Can you work these out from the model? Positions are in its coordinate system, mm. A direction names the side the tool comes from. Round coordinates to 2 decimals unless told otherwise and drop trailing zeros. Loops run counter-clockwise (first coordinate to the right, second up) from the corner with the lowest first, then second, coordinate; pieces in that order, holes last. Notation, with made-up numbers: M 41.5,-4.5 L 61.5,-4.5 A24 ccw 61.5,16.5 Z; hole C 85.5,-2 d9. An arc over 180 degrees is marked long. Return JSON: item names as keys, results as strings.
Autodesk Inventor part; units mm, degrees
ref_plane "YZ Plane" through (0, 0, 0) normal (1, 0, 0) x (0, 1, 0)
ref_plane "XZ Plane" through (0, 0, 0) normal (0, 1, 0) x (-1, 0, 0)
ref_plane "XY Plane" through (0, 0, 0) normal (0, 0, 1) x (1, 0, 0)
sketch "Esquisse1" plane through (0, 0, 0) normal (0, 0, 1) x (1, 0, 0)
  circle A0 centre (0, 0) radius 3
  dimension "d0" = 6
extrude "Extrusion1" add sketch "Esquisse1" along normal blind 36.5
sketch "Esquisse2" plane through (0, 0, 36.5) normal (0, 0, 1) x (1, 0, 0)
  circle A0 centre (0, 0) radius 2.5
  dimension "d3" = 5
extrude "Extrusion2" add sketch "Esquisse2" along normal blind 3
sketch "Esquisse3" plane through (0, 0, 0) normal (0, 0, -1) x (-1, 0, 0)
  circle A0 centre (0, 0) radius 2.5
  dimension "d6" = 5
extrude "Extrusion3" add sketch "Esquisse3" along normal blind 12
sketch "Esquisse4" plane through (0, 0, -12) normal (0, 0, -1) x (-1, 0, 0)
  circle A0 centre (0, 0) radius 2
  dimension "d9" = 4
extrude "Extrusion4" add sketch "Esquisse4" along normal blind 29
thread "Filetage1"
fillet "Congé1" radius 0.5 1 edges at (2, 0, -41)
properties part number "AxeArriere" material "Acier inoxydable"
Q1. On a 3-axis mill with a long thin cutter (end or side, diameter ignored), from which of +Z, -Z, +X, -X, +Y, -Y can I reach the whole of each face in a straight line? I mean faces 1 (the flat face through (0, 0, -41)), 2 (the cylindrical face through (0.54, 2.44, -5.92)), 3 (the cylindrical face through (-0.54, 2.44, 37.98)). Say none if no direction works.
Results:
{"face 1": "-Z, +X, -X, +Y, -Y", "face 2": "-Z", "face 3": "+Z"}
Q2. Suppose I cut it at C-C, the plane z = -1. Please give me the cut outline in (x, y), plus the area to 3 significant figures.
Results:
{"outline": "C 0,0 d5", "area": "19.6 mm2"}
Q3. Suppose I cut it at D-D, the plane z = -19. Please give me the cut outline in (x, y), plus the area to 3 significant figures.
Results:
{"outline": "C 0,0 d4", "area": "12.6 mm2"}
Q4. If I drill on line 1 along Z through (x, y) = (-0.85, -2.65); line 2 along Z through (x, y) = (1.15, 1.75); line 3 along X through (y, z) = (0.1, 11), over which ranges is the centre line in solid material (lowest first)?
Results:
{"line 1": "z = 0 to 36.5", "line 2": "z = -12 to 39.5", "line 3": "x = -3 to 3"}
Q5. I'm going to push flat-ended pins straight in: pin 1 Ø1.5 at (y, z) = (2, 7.5) entering from +X; pin 2 Ø1 at (x, z) = (0, -22.5) entering from +Y. Where does each tip first touch, or does it pass through?
Results:
{"pin 1": "stops at x = 2.73", "pin 2": "stops at y = 2"}
Q6. Suppose I cut it at A-A, the plane x = 0. Please give me the cut outline in (y, z), plus the area to 3 significant figures.
Results:
{"outline": "M -3,0 L -2.5,0 L -2.5,-12 L -2,-12 L -2,-40.5 A0.5 ccw -1.5,-41 L 1.5,-41 A0.5 ccw 2,-40.5 L 2,-12 L 2.5,-12 L 2.5,0 L 3,0 L 3,36.5 L 2.5,36.5 L 2.5,39.5 L -2.5,39.5 L -2.5,36.5 L -3,36.5 Z", "area": "410 mm2"}
